Input: part model. Units: mm. Frame: model coordinates. Give positions to 0.01 mm unless a question says otherwise; leave off trailing zeros. Order: outer loops, then holes, each group sorted by start corner. A loop starts at its lowest first (then second) coordinate and runs counter-clockwise, first axis right, second up. Notation, with made-up numbers: (19, 2.5) - (60, 2.5) arc R23 ccw to (60, 20.5) - close; hole circle Ø9 at (72, 43). An arc over 180 degrees is marked (long way). Answer in a Markdown table with one row per item. Add a question column.
1. Contact query for flat-ended pins moving along their axis: pin 1 (2 mm diameter, centred on x = 3, y = -1, fed in from +Z); pin 2 (1 mm diameter, centred on x = 1.5, z = -1, fed in from -Y). Output: stop coordinate, or through.
2. Ray query, line 1 (Y direction, x = 7, z = 0.1); line 2 (Z direction, x = -6.5, y = -1.2); line 3 (Z direction, x = 5.5, y = -2.4). Return the intervals inside material, ascending. Write a range as [from, to].
3. Section query B-B on x = -2.5. Return loops of the section in (y, z).
Autodesk Fusion 360 part; units mm, degrees
sketch "Sketch1" plane through (0, 0, 0) normal (1, 0, 0) x (0, 1, 0)
  circle A0 centre (0, 0) radius 2.75
  line L0 (0, 0) -> (0, 2.75) construction
  line L1 (0, 0) -> (0, -2.75) construction
  line L2 (0, 2.75) -> (1.5, 2.75)
  line L3 (1.5, 2.75) -> (1.5, -2.75)
  line L4 (1.5, -2.75) -> (0, -2.75)
  line L5 (0, -2.75) -> (0, 2.75)
  dimension "d1" = 5.5
  dimension "d42" = 1.5
extrude "Extrude1" add sketch "Sketch1" along normal mid plane 15.4 contours A0 L5 | A0 L3 L5 | A0 L3
ref_plane "WorkPlane1" through (-7.5, 0, 0) normal (-1, 0, 0) x (0, -1, 0)
ref_plane "WorkPlane2" through (0, 0, 0) normal (1, 0, 0) x (0, 1, 0)
ref_plane "WorkPlane3" through (3.85, 0, 0) normal (1, 0, 0) x (0, 1, 0)
ref_plane "WorkPlane4" through (5.775, 0, 0) normal (1, 0, 0) x (0, 1, 0)
ref_plane "WorkPlane5" through (1.925, 0, 0) normal (1, 0, 0) x (0, 1, 0)
ref_plane "WorkPlane6" through (-3.85, 0, 0) normal (-1, 0, 0) x (0, -1, 0)
ref_plane "WorkPlane7" through (-5.775, 0, 0) normal (-1, 0, 0) x (0, -1, 0)
ref_plane "WorkPlane8" through (-1.925, 0, 0) normal (-1, 0, 0) x (0, -1, 0)
sketch "Sketch3" plane through (0, 0, 0) normal (1, 0, 0) x (0, 1, 0)
  circle A0 centre (0, 0) radius 2.75
  circle A1 centre (0, 0) radius 2.625
  dimension "d12" = 5.5
  dimension "d13" = 5.25
extrude "Extrude2" cut sketch "Sketch3" along normal mid plane 0.25
sketch "Sketch4" plane through (-7.5, 0, 0) normal (-1, 0, 0) x (0, 1, 0)
  circle A0 centre (0, 0) radius 2.75
  circle A1 centre (0, 0) radius 2.625
  dimension "d16" = 5.5
  dimension "d17" = 5.25
sketch "Sketch5" plane through (-1.925, 0, 0) normal (-1, 0, 0) x (0, 1, 0)
  circle A0 centre (0, 0) radius 2.75
  circle A1 centre (0, 0) radius 2.625
  dimension "d18" = 5.5
  dimension "d19" = 5.25
extrude "Extrude3" cut sketch "Sketch5" along normal mid plane 0.25
sketch "Sketch6" plane through (-3.85, 0, 0) normal (-1, 0, 0) x (0, 1, 0)
  circle A0 centre (0, 0) radius 2.75
  circle A1 centre (0, 0) radius 2.625
  dimension "d22" = 5.5
  dimension "d23" = 5.25
extrude "Extrude4" cut sketch "Sketch6" along normal mid plane 0.25
sketch "Sketch7" plane through (-5.775, 0, 0) normal (-1, 0, 0) x (0, 1, 0)
  circle A0 centre (0, 0) radius 2.75
  circle A1 centre (0, 0) radius 2.625
  dimension "d26" = 5.5
  dimension "d27" = 5.25
extrude "Extrude5" cut sketch "Sketch7" along normal mid plane 0.25
sketch "Sketch8" plane through (1.925, 0, 0) normal (1, 0, 0) x (0, 1, 0)
  circle A0 centre (0, 0) radius 2.75
  circle A1 centre (0, 0) radius 2.625
  dimension "d30" = 5.5
  dimension "d31" = 5.25
extrude "Extrude6" cut sketch "Sketch8" along normal mid plane 0.25
sketch "Sketch9" plane through (3.85, 0, 0) normal (1, 0, 0) x (0, 1, 0)
  circle A0 centre (0, 0) radius 2.75
  circle A1 centre (0, 0) radius 2.625
  dimension "d34" = 5.5
  dimension "d35" = 5.25
extrude "Extrude7" cut sketch "Sketch9" along normal mid plane 0.25
sketch "Sketch10" plane through (5.775, 0, 0) normal (1, 0, 0) x (0, 1, 0)
  circle A0 centre (0, 0) radius 2.75
  circle A1 centre (0, 0) radius 2.625
  dimension "d38" = 5.5
  dimension "d39" = 5.25
extrude "Extrude8" cut sketch "Sketch10" along normal mid plane 0.25
extrude "Extrude9" add sketch "Sketch1" along normal mid plane 15.4 contours A0 L2 L3 | A0 L3 L5 | A0 L3 L4
extrude "Extrude10" cut sketch "Sketch1" along normal mid plane 20 contours A0 L3
Answer:
| question | item | result |
|---|---|---|
| 1 | pin 1 | stops at z = 2.75 |
| 1 | pin 2 | stops at y = -2.7 |
| 2 | line 1 | y = [-2.75, 1.5] |
| 2 | line 2 | z = [-2.47, 2.47] |
| 2 | line 3 | z = [-1.34, 1.34] |
| 3 | outline | (0, -2.75) - (1.5, -2.75) - (1.5, 2.75) - (0, 2.75) arc R2.75 ccw to start |
